Job drawing, mm, ordinate dimensions from the low corner. One solid piece. A direction names the side the tool comes from. Round coordinates to 2 decimals unless told otherwise and drop trailing zeros. Loops run counter-clockwise (first coordinate to the right, second up) from the corner with the lowest first, then second, coordinate; pieces in that order, holes last.
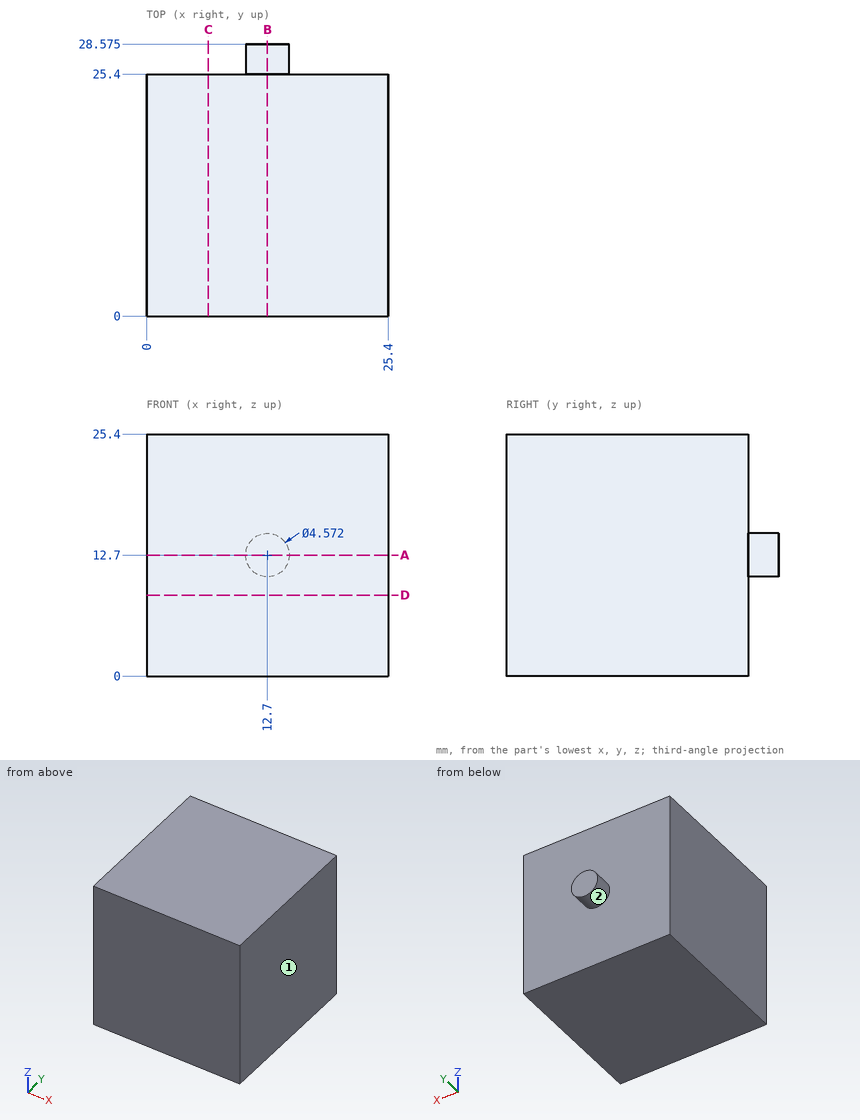
(1) Which spindle directions (+Z, -Z, +X, -X, +Y, -Y) get a long thin tool onto all of the face, cutting with end or side? Do the marked faces 1 and 2. Say none if no direction does.
Responses:
face 1: +Z, -Z, +X, +Y, -Y
face 2: +Y
(2) Slice it at A-A on z = 12.7. List the corners of the cut face in (x, y) (3 decimals).
Responses:
outline: (0, 0) - (25.4, 0) - (25.4, 25.4) - (14.986, 25.4) - (14.986, 28.575) - (10.414, 28.575) - (10.414, 25.4) - (0, 25.4) - close
(3) Slice it at B-B on x = 12.7. List the corners of the cut face in (y, z) (3 decimals).
Responses:
outline: (0, 0) - (25.4, 0) - (25.4, 10.414) - (28.575, 10.414) - (28.575, 14.986) - (25.4, 14.986) - (25.4, 25.4) - (0, 25.4) - close
(4) Slice it at C-C on x = 6.5. List the corners of the cut face in (y, z).
Responses:
outline: (0, 0) - (25.4, 0) - (25.4, 25.4) - (0, 25.4) - close
(5) Probe line 1 (Y direction, x = 2.75, z = 16.75); line 2 (Z direction, x = 13.75, y = 25.75); line 3 (Z direction, x = 11.25, y = 26.75). List the from-to ranges inside material, lowest first.
Responses:
line 1: y = 0 to 25.4
line 2: z = 10.67 to 14.73
line 3: z = 10.93 to 14.47
